Verification items for this drawing (mm, ordinates from the low corner). A direction names the side the tool comes from. Give positions to 0.01 mm unless a question says otherwise; leave off trailing zeros. Loops run counter-clockwise (first coordinate to the right, second up) from the corner with the lowest first, then second, coordinate; pieces in that order, holes last. Notation, with made-up numbers: (23, 88) -> (42, 88) arc R9 ccw to (42, 103) -> close; hole circle Ø1 at (82.25, 44). An arc over 180 degrees is marked (long way). Answer in a Markdown table with one row per item. Add a question column.
Q1. Section check D-D on z = 17.75. Enter the section's corners in (x, y), and give its area (3 significant figures).
Q2. Section check C-C on z = 12.25. Enter the section's corners in (x, y).
Q3. Section check A-A on x = 1.5. Enter the section's corners in (y, z).
Q4. Material ranges on probe 1 along Z at (x, y) = (1.95, 2.85); probe 2 along X at (y, z) = (2.2, 8); probe 3 along X at (y, z) = (2.05, 16.75), recorded low to high.
Q5. Set-up check for the marked faces 4 and 5: record each of +Z, -Z, +X, -X, +Y, -Y from which the full face is reachable in a straight line by a thin tool's end or side.
Q6. Release check for a two-part mould opening along Z. For the marked faces 1, 2 and 3 record: pulls with the +Z half, pulls with the -Z half, needs draft (parallel to the pull), parting line crosses it, or undercut.
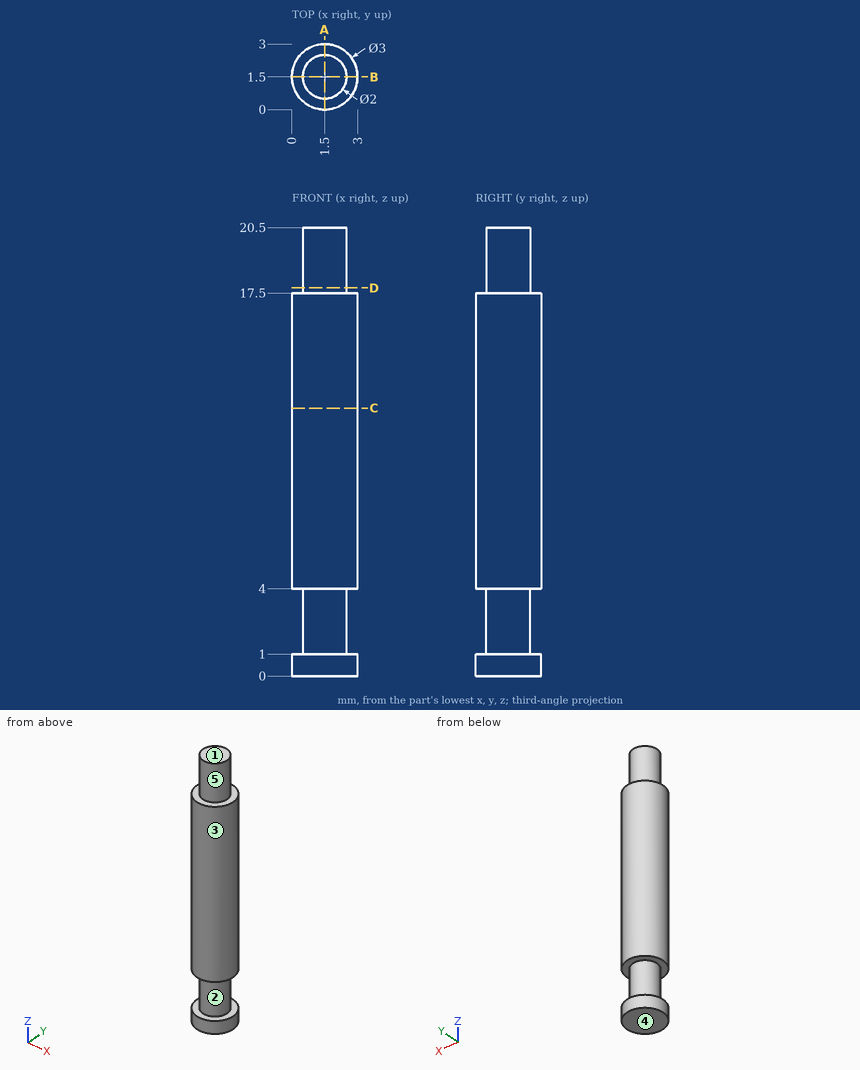
Taken from the geometry:
| question | item | result |
|---|---|---|
| 1 | outline | circle Ø2 at (1.5, 1.5) |
| 1 | area | 3.14 mm² |
| 2 | outline | circle Ø3 at (1.5, 1.5) |
| 3 | outline | (0, 0) -> (3, 0) -> (3, 1) -> (2.5, 1) -> (2.5, 4) -> (3, 4) -> (3, 17.5) -> (2.5, 17.5) -> (2.5, 20.5) -> (0.5, 20.5) -> (0.5, 17.5) -> (0, 17.5) -> (0, 4) -> (0.5, 4) -> (0.5, 1) -> (0, 1) -> close |
| 4 | probe 1 | z = 0 to 1, 4 to 17.5 |
| 4 | probe 2 | x = 0.17 to 2.83 |
| 4 | probe 3 | x = 0.1 to 2.9 |
| 5 | face 4 | -Z, +X, -X, +Y, -Y |
| 5 | face 5 | +Z |
| 6 | face 1 | pulls with the +Z half |
| 6 | face 2 | undercut |
| 6 | face 3 | needs draft |
